```python
from build123d import *

# Parameters (mm, degrees)
F1_DEPTH = 50


with BuildPart() as f1:
    # F0 (on Top) → F1 (new body)
    with BuildSketch(Plane.XY):
        Polygon((-3, 42), (-3, -3), (30.740852, -3), (38, -3), (38, 8), (38, 42), (17.5, 42), align=None)
        with BuildLine():
            Line((35, 21.5), (35, 8))
            ThreePointArc((35, 8), (33.112912, 3.870902), (30.740852, 0))
            Line((30.740852, 0), (4.259148, 0))
            ThreePointArc((4.259148, 0), (1.887088, 3.870902), (0, 8))
            Line((0, 8), (0, 21.5))
            ThreePointArc((0, 21.5), (17.5, 39), (35, 21.5))
        make_face(mode=Mode.SUBTRACT)
    extrude(amount=F1_DEPTH)


solid = f1.part
```
CAD build for the part. Positions are in the model's coordinates, mm. A direction names the side the tool comes from. Round coordinates to 2 decimals unless told otherwise and drop trailing zeros. Order: outer loops, then holes, each group sorted by start corner. A loop starts at its lowest first (then second) coordinate and runs counter-clockwise, first axis right, second up.
Q1. Slice it at A-A (y = 15). Write the cut outline in (x, z), and give its area (3 significant figures).
Q2. Wall check: L1, parallel to X at y = 17.5, z = 39.5; L2, parallel to Y at x = 10.5, z = 26.5; L3, parallel to X at y = 27, z = 22.5. Give the ranges that are in metal, low to high.
Q3. Two-plate mould, pull along Y, no slides. Class faces 3 (the flat face through (35.4, 19.8, 0)), 4 (the flat face through (18, 42, 25)), 5 (the flat face through (35, 15, 25)): pulls with the +Y half, pulls with the -Y half, needs draft (parallel to the pull), parting line crosses it, or undercut.
Q4. Which spindle directions (+Z, -Z, +X, -X, +Y, -Y) get a long thin tool onto all of the face, cutting with end or side? Do faces 1 (the flat face through (38, 19, 25)), 2 (the cylindrical face through (17.115, 38.996, 24.65)). Say none if no direction does.
Q5. Drop a flat-ended pin along its axis: pin 1 (2 mm diameter, centred on x = 14.5, y = 37.5, fed in from -Z). Give the stop position or say it passes through.
Q6. Slice it at B-B (x = 17.5). Write the cut outline in (y, z).
Q7. Slice it at C-C (z = 42.5). Write the cut outline in (x, y).
Results below:
1. outline: (-3, 0) - (0, 0) - (0, 50) - (-3, 50) - close; (35, 0) - (38, 0) - (38, 50) - (35, 50) - close
1. area: 300 mm2
2. L1: x = -3 to 0, 35 to 38
2. L2: y = -3 to 0, 37.54 to 42
2. L3: x = -3 to 0.89, 34.11 to 38
3. face 3: needs draft
3. face 4: pulls with the +Y half
3. face 5: undercut
4. face 1: +Z, -Z, +X, +Y, -Y
4. face 2: +Z, -Z
5. pin 1: passes through
6. outline: (-3, 0) - (0, 0) - (0, 50) - (-3, 50) - close; (39, 0) - (42, 0) - (42, 50) - (39, 50) - close
7. outline: (-3, -3) - (38, -3) - (38, 42) - (-3, 42) - close; hole (0, 8) arc R37.51 ccw to (4.26, 0) - (30.74, 0) arc R37.51 ccw to (35, 8) - (35, 21.5) arc R17.5 ccw to (0, 21.5) - close
